Build history of the part. All positions in model axes, mm. A direction names the side the tool comes from. Coordinates: 2 decimals unless noted, no trailing zeros. Loops run counter-clockwise (first coordinate to the right, second up) from the corner with the lowest first, then second, coordinate; pieces in that order, holes last. Notation, with made-up numbers: (13, 78.25) - (36, 78.25) arc R18 cw to (36, 86.25) - close; hole circle Ø10 at (-30, 81). An arc over 180 degrees is marked (long way). One line per item, written item: value.
Autodesk Inventor part; units mm, degrees
ref_plane "YZ Plane" through (0, 0, 0) normal (1, 0, 0) x (0, 1, 0)
ref_plane "XZ Plane" through (0, 0, 0) normal (0, 1, 0) x (-1, 0, 0)
ref_plane "XY Plane" through (0, 0, 0) normal (0, 0, 1) x (1, 0, 0)
sketch "Sketch1" plane through (0, 0, 0) normal (0, 1, 0) x (-1, 0, 0)
  line L0 (-9.7302, 52.2849) -> (-85.9302, 52.2849)
  line L1 (-85.9302, 52.2849) -> (-85.9302, -100.1151)
  line L2 (-85.9302, -100.1151) -> (-9.7302, -100.1151)
  line L3 (-9.7302, -100.1151) -> (-9.7302, 52.2849)
  point P0 (0, 0)
  dimension "d0" = 152.4
  dimension "d1" = 76.2
extrude "Plate1" add sketch "Sketch1" along normal blind 3.048
sketch "Sketch2" plane through (12.7782, 0, 52.2849) normal (-1, 0, 0) x (0, -1, 0)
  line L0 (0, -152.4) -> (0, 0)
  line L1 (0, 0) -> (-152.4, 0)
  line L2 (-152.4, 0) -> (-152.4, -152.4)
  line L3 (-152.4, -152.4) -> (0, -152.4)
edge flange "Flange1" height 152.4 angle 90 thickness 3.048 bend radius 3.048 thickness toward (-1, 0, 0) relief tear relief width 3.048 relief depth 1.524 edges at (9.7302, 3.048, -23.9151) wall of the first edge with corners at (12.7782, 0, -100.1151) (12.7782, 0, 52.2849) (12.7782, 152.4, 52.2849) (12.7782, 152.4, -100.1151)
bend "Bend1"
corner "Corner1"
sketch "Sketch5" plane through (12.7782, 152.4, 52.2849) normal (1, 0, 0) x (0, 0, -1)
  circle A0 centre (57.15, -76.2) radius 38.1
  line L0 (0, -152.4) -> (152.4, -152.4)
  line L1 (152.4, 0) -> (152.4, -146.304)
  point P0 (52.2849, -152.4)
  dimension "d23" = 76.2
  dimension "d24" = 76.2
  dimension "d25" = 95.25
extrude "Cut1" cut sketch "Sketch5" against normal blind 3.048
sketch "Sketch6" plane through (12.7782, 152.4, 52.2849) normal (1, 0, 0) x (0, 0, -1)
  circle A0 centre (57.15, -76.2) radius 38.1
  line L0 (19.05, -76.2) -> (19.05, 0)
  line L1 (152.4, 0) -> (0, 0)
  line L2 (19.05, 0) -> (31.75, 0)
  line L3 (31.75, 0) -> (31.75, -47.8019)
  arc A1 (31.75, -47.8019) -> (19.05, -76.2) centre (57.15, -76.2) ccw
  point P0 (52.2849, -152.4)
  dimension "d47" = 12.7
extrude "Cut2" cut sketch "Sketch6" against normal blind 3.048 contours A0 L0 L1 L3
sketch "Sketch7" plane through (12.7782, 149.352, 33.2349) normal (0, 1, 0) x (-1, 0, 0)
  line L0 (0, 19.05) -> (0, 0)
  line L1 (0, 0) -> (44.45, 0)
  line L2 (44.45, 0) -> (44.45, 19.05)
  line L3 (44.45, 19.05) -> (0, 19.05)
edge flange "Flange3" height 44.45 angle 90 thickness 3.048 bend radius 3.048 thickness toward (0, 1, 0) relief tear relief width 3.048 relief depth 1.524 corner gap 3.048 corner form 0 edges at (9.7302, 152.4, 42.7599) (9.7302, 152.4, -39.7901) wall of the first edge with corners at (12.7782, 149.352, 52.2849) (12.7782, 149.352, 33.2349) (-31.6718, 149.352, 33.2349) (-31.6718, 149.352, 52.2849)
bend "Bend3"
corner "Corner3"
sketch "Sketch8" plane through (-31.6718, 152.4, 20.5349) normal (0, 1, 0) x (1, 0, 0)
  circle A0 centre (19.05, 95.25) radius 6.35
  circle A1 centre (19.05, 25.4) radius 6.35
  line L0 (38.354, 0) -> (0, 0)
  line L1 (0, 0) -> (0, 120.65)
  point P0 (31.6718, 20.5349)
  dimension "d40" = 12.7
  dimension "d41" = 69.85
  dimension "d42" = 25.4
  dimension "d43" = 19.05
  dimension "d44" = 19.05
extrude "Cut3" cut sketch "Sketch8" against normal blind 3.048
sketch "Sketch9" plane through (-31.6718, 152.4, 52.2849) normal (0, 1, 0) x (1, 0, 0)
  circle A0 centre (19.05, 9.525) radius 4.7625
  line L0 (38.354, 0) -> (0, 0)
  line L1 (0, 0) -> (0, 19.05)
  point P0 (31.6718, 52.2849)
  dimension "d48" = 9.525
  dimension "d49" = 9.525
  dimension "d50" = 19.05
extrude "Cut4" cut sketch "Sketch9" against normal blind 3.048
sketch "Sketch10" plane through (-31.6718, 149.352, 20.5349) normal (0, 0, 1) x (1, 0, 0)
  point P0 (31.6718, -149.352)
sketch "Sketch11" plane through (0, 3.048, 0) normal (0, 1, 0) x (1, 0, 0)
  circle A0 centre (66.8802, -42.7599) radius 3.175
  circle A1 centre (28.7802, -42.7599) radius 3.175
  line L0 (85.9302, -52.2849) -> (15.8262, -52.2849)
  line L1 (85.9302, 100.1151) -> (85.9302, -52.2849)
  circle A2 centre (66.8802, 90.5901) radius 3.175
  circle A3 centre (28.7802, 90.5901) radius 3.175
  line L2 (15.8262, 100.1151) -> (85.9302, 100.1151)
  point P0 (0, 0)
  dimension "d53" = 6.35
  dimension "d54" = 6.35
  dimension "d55" = 9.525
  dimension "d56" = 9.525
  dimension "d57" = 38.1
  dimension "d58" = 19.05
  dimension "d59" = 6.35
  dimension "d60" = 6.35
  dimension "d63" = 38.1
  dimension "d65" = 9.525
  dimension "d66" = 9.525
  dimension "d67" = 19.05
extrude "Cut5" cut sketch "Sketch11" against normal blind 3.048
equation "\"d26\" = Thickness"
equation "\"d28\" = Thickness"
equation "\"d45\" = Thickness"
equation "\"d51\" = Thickness"
equation "\"d68\" = Thickness"
equation "\"d3\" = BendReliefWidth"
equation "\"d4\" = BendReliefDepth"
equation "\"d5\" = MinimumRemnant"
equation "\"d6\" = BendRadius"
equation "\"d9\" = BendRadius"
equation "\"d10\" = CornerReliefSize"
equation "\"d11\" = GapSize"
equation "\"d12\" = JacobiRadiusSize"
equation "\"d30\" = BendReliefWidth"
equation "\"d31\" = BendReliefDepth"
equation "\"d32\" = MinimumRemnant"
equation "\"d33\" = BendRadius"
equation "\"d36\" = BendRadius"
equation "\"d37\" = CornerReliefSize"
equation "\"d38\" = GapSize"
equation "\"d39\" = JacobiRadiusSize"
equation "\"BendRadius\" = Thickness"
equation "\"BendReliefWidth\" = Thickness"
equation "\"BendReliefDepth\" = 0.5 * Thickness"
equation "\"CornerReliefSize\" = 4 * Thickness"
equation "\"MinimumRemnant\" = 2 * Thickness"
equation "\"TransitionRadius\" = BendRadius"
equation "\"JacobiRadiusSize\" = BendRadius"
equation "\"GapSize\" = Thickness"
equation "\"d2\" = BendRadius"
properties part number "Tape Measure Dispenser Part 2"
Item 1: Cut at B-B, the plane z = -58. Write the cut outline in (x, y), then the cut area to 3 significant figures.
Check result:
outline: (-31.67, 149.35) - (6.68, 149.35) arc R3.05 cw to (9.73, 146.3) - (9.73, 6.1) arc R6.1 ccw to (15.83, 0) - (85.93, 0) - (85.93, 3.05) - (15.83, 3.05) arc R3.05 cw to (12.78, 6.1) - (12.78, 146.3) arc R6.1 ccw to (6.68, 152.4) - (-31.67, 152.4) - close
area: 802 mm^2
Item 2: Cut at D-D, the plane z = -24. Write the cut outline in (x, y).
Check result:
outline: (-31.67, 149.35) - (6.68, 149.35) arc R3.05 cw to (9.73, 146.3) - (9.73, 109.15) - (12.78, 109.15) - (12.78, 146.3) arc R6.1 ccw to (6.68, 152.4) - (-31.67, 152.4) - close; (9.73, 6.1) arc R6.1 ccw to (15.83, 0) - (85.93, 0) - (85.93, 3.05) - (15.83, 3.05) arc R3.05 cw to (12.78, 6.1) - (12.78, 43.25) - (9.73, 43.25) - close
Item 3: Pull direction X, two halves, no side cores. Call faces 4 (the face through (9.73, 93, -40)), 5 (the face through (51, 3.048, -23)), 6 (the face through (66.19, 1.55, 45.86)), 7 (the face through (-6.565, 150.897, -6.772)): released by +X, released by -X, zero draft, split by the parting line, or undercut.
Check result:
face 4: released by -X
face 5: zero draft
face 6: undercut
face 7: undercut
Item 4: Tool access for faces 1 (the face through (-8, 149.352, 45)), 2 (the face through (63.71, 1.55, -90.73)), 3 (the face through (10, 126, 33.235)): list every direction of +Z, -Z, +X, -X, +Y, -Y with a clear straight run to the whole face (end or side of a thin tool).
Check result:
face 1: +Z, -Z, -X, -Y
face 2: +Y, -Y
face 3: +X, -X, +Y
Item 5: Cut at A-A, the plane y = 125. Write the cut outline in (x, z), then the cut area to 3 significant figures.
Check result:
outline: (9.73, -100.12) - (12.78, -100.12) - (12.78, 20.53) - (9.73, 20.53) - close; (9.73, 33.23) - (12.78, 33.23) - (12.78, 52.28) - (9.73, 52.28) - close
area: 426 mm^2
Item 6: Probe probe 1 along Z at (x, y) = (10.45, 76.2); probe 2 along Y at (x, z) = (6, -72); probe 3 along Y at (x, z) = (18, -13). List the from-to ranges inside material, lowest first. Write a range as from..to.
Check result:
probe 1: z = -100.12..-42.97, 33.23..52.28
probe 2: y = 149.35..152.4
probe 3: y = 0..3.05
Item 7: Drop flat-ended pins along their axis: P1, Ø12, axis at x = 3.5, z = -51.5, coming from the -Y side; P2, Ø11.5, axis at x = -12.62, z = -4.87, coming from the +Y side; P3, Ø12, axis at y = 114.5, z = -13, coming from the -X side; P4, Ø19, axis at x = -18.5, z = -65.5, coming from the -Y side. Give the stop position or say it passes through.
Check result:
P1: stops at y = 147.47
P2: passes through
P3: stops at x = 9.73
P4: stops at y = 149.35
Item 8: Cut at C-C, the plane y = 107. Write the cut outline in (x, z), then the cut area to 3 significant figures.
Check result:
outline: (9.73, -100.12) - (12.78, -100.12) - (12.78, -27.29) - (9.73, -27.29) - close; (9.73, 17.56) - (12.78, 17.56) - (12.78, 20.53) - (9.73, 20.53) - close; (9.73, 33.23) - (12.78, 33.23) - (12.78, 52.28) - (9.73, 52.28) - close
area: 289 mm^2
